from build123d import *

# Parameters (mm, degrees)
SKETCH2_R           = 11
BOSS_EXTRUDE1_DEPTH = 5.25
CHAMFER1_SIZE       = 0.5


with BuildPart() as part:
    # Sketch2 → Boss-Extrude1 (new body, symmetric)
    with BuildSketch(Plane.XY):
        Circle(SKETCH2_R)
    extrude(amount=BOSS_EXTRUDE1_DEPTH, both=True)

    # Sketch4 → Cut-Revolve1 (revolve, cut)
    with BuildSketch(Plane(origin=(0, 0, 0), x_dir=(0, 0, -1), z_dir=(1, 0, 0))):
        with BuildLine():
            Line((7, -6.45), (7, 0))
            Line((7, 0), (-7, 0))
            Line((-7, 0), (-7, -6.45))
            ThreePointArc((-7, -6.45), (0, -9.518534551), (7, -6.45))
        make_face()
    revolve(axis=Axis((0, 0, -7), (0, 0, 1)), mode=Mode.SUBTRACT)

    # Chamfer1
    chamfer1_edges = [part.edges().sort_by_distance(p)[0] for p in [
        (-11, 0, -5.25),
        (-11, 0, 5.25),
    ]]
    chamfer(chamfer1_edges, length=CHAMFER1_SIZE)


solid = part.part
Geometry check sheet. Reference: the model listing, model coordinates, mm. Coordinates: 2 decimals unless noted, no trailing zeros. Write each loop counter-clockwise with the first axis right and the second up, starting at its lowest first coordinate (ties: lowest second). Pieces come first, ordered by that corner, then holes. Notation, with made-up numbers: (-0.75, 1) -> (54.25, 1) arc R20 cw to (54.25, 31) -> close; hole circle Ø11 at (82, 48.5). An arc over 180 degrees is marked (long way). One line per question, with ' | ' between items.
1. Cross-section at A-A on y = 0. Record the cut outline in (x, z), and give its area (3 significant figures).
Answers:
outline: (-11, -4.75) -> (-10.5, -5.25) -> (-7.94, -5.25) arc R9.52 cw to (-7.94, 5.25) -> (-10.5, 5.25) -> (-11, 4.75) -> close; (7.94, -5.25) -> (10.5, -5.25) -> (11, -4.75) -> (11, 4.75) -> (10.5, 5.25) -> (7.94, 5.25) arc R9.52 cw to start | area: 41.3 mm²
2. Depth check by flat-ended pin: pin 1 Ø2 at (y, z) = (-2.5, 3.5) entering from -X; pin 2 Ø4 at (y, z) = (-8, -1.5) entering from -X; pin 3 Ø1.5 at (y, z) = (-2.5, 2.5) entering from +X. Enter the tip coordinate at first touch or a pass-through.
Answers:
pin 1: stops at x = -10.9 | pin 2: stops at x = -9.22 | pin 3: stops at x = 10.86
3. Thickness scan on probe 1 along X at (y, z) = (-4.75, -1); probe 2 along X at (y, z) = (3, -2.5); probe 3 along Z at (x, y) = (6, -6.5). Record the ranges inside material, lowest first. Write a range as from..to.
Answers:
probe 1: x = -9.92..-8.19, 8.19..9.92 | probe 2: x = -10.58..-8.68, 8.68..10.58 | probe 3: z = -5.25..-3.51, 3.51..5.25
4. Cross-section at C-C on z = 3.5. Record the cut outline in (x, y).
Answers:
outline: circle Ø22 at (0, 0); hole circle Ø17.7 at (0, 0)
5. Cross-section at D-D on z = -1. Record the cut outline in (x, y), and give its area (3 significant figures).
Answers:
outline: circle Ø22 at (0, 0); hole circle Ø18.93 at (0, 0) | area: 98.6 mm²
